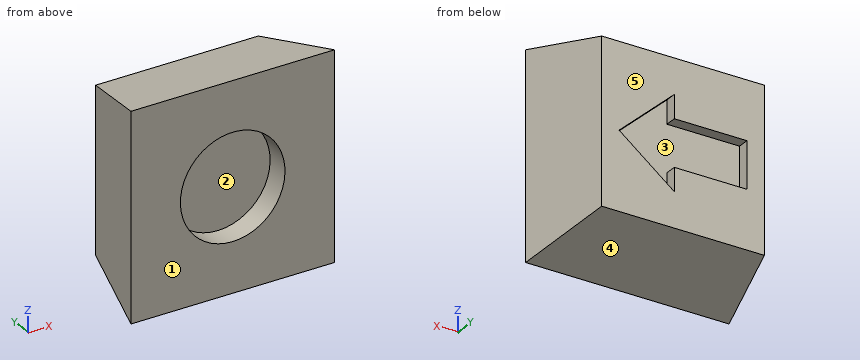
from build123d import *

# Parameters (mm, degrees)
SKETCH1_W           = 7
SKETCH1_H           = 7
BOSS_EXTRUDE1_DEPTH = 3
CUT_EXTRUDE1_DEPTH  = 7
CUT_EXTRUDE2_DEPTH  = 11
SKETCH4_R           = 1.8
CUT_EXTRUDE3_DEPTH  = 0.8
SKETCH5_W           = 2.5
SKETCH5_H           = 1.6
CUT_EXTRUDE4_DEPTH  = 0.4


with BuildPart() as part:
    # Sketch1 → Boss-Extrude1 (new body)
    with BuildSketch(Plane(origin=(0, 0, 0), x_dir=(1, 0, 0), z_dir=(0, 1, 0))):
        with Locations((3.5, 3.5)):
            Rectangle(SKETCH1_W, SKETCH1_H)
    extrude(amount=BOSS_EXTRUDE1_DEPTH)

    # Sketch2 → Cut-Extrude1 (cut)
    with BuildSketch(Plane.XY):
        Polygon((0, 0), (0.7, 3), (0, 3), align=None)
        Polygon((7, 0), (6.3, 3), (7, 3), align=None)
    extrude(amount=-CUT_EXTRUDE1_DEPTH, mode=Mode.SUBTRACT)

    # Sketch3 → Cut-Extrude2 (cut)
    with BuildSketch(Plane(origin=(0, 0, 0), x_dir=(0, 0, -1), z_dir=(1, 0, 0))):
        Polygon((0, 0), (0.7, 3), (0, 3), align=None)
        Polygon((7, 3), (6.3, 3), (7, 0), align=None)
    extrude(amount=CUT_EXTRUDE2_DEPTH, mode=Mode.SUBTRACT)

    # Sketch4 → Cut-Extrude3 (cut)
    with BuildSketch(Plane.XZ):
        with Locations(Location((3.5, -3.5, 0), (0, 0, 270))):
            Circle(SKETCH4_R)
    extrude(amount=-CUT_EXTRUDE3_DEPTH, mode=Mode.SUBTRACT)

    # Sketch5 → Cut-Extrude4 (cut)
    with BuildSketch(Plane(origin=(0, 3, 0), x_dir=(1, 0, 0), z_dir=(0, 1, 0))):
        with Locations((2.55, 3.5)):
            Rectangle(SKETCH5_W, SKETCH5_H)
        Polygon((3.8, 1.9), (3.8, 2.7), (3.8, 4.3), (3.8, 5.1), (5.7, 3.624818901), align=None)
    extrude(amount=-CUT_EXTRUDE4_DEPTH, mode=Mode.SUBTRACT)


solid = part.part
Read the model definition and answer for the solid it produces. Units are mm, in the model's axes. Face numbers are marked on the shaded views. A direction names the side the tool comes from. Round coordinates to 2 decimals unless told otherwise and drop trailing zeros. Write each loop counter-clockwise with the first axis right and the second up, starting at its lowest first coordinate (ties: lowest second). Pieces come first, ordered by that corner, then holes. Notation, with made-up numbers: (-33.5, 20) - (6.5, 20) arc R25 ccw to (6.5, 41) - close; hole circle Ø9 at (33.5, 18.25). An arc over 180 degrees is marked (long way). One line per question, with ' | ' between items. Start each with the question number.
1. Find the intervals of material crossed by probe 1 along X at (y, z) = (0.3, -4); probe 2 along Z at (x, y) = (2, 0.55); probe 3 along Y at (x, z) = (2.25, -2.5), in increasing order. Write a range as [from, to].
2. Section D-D (x = 5.5) is taken. Determine the outline of the cut face in (y, z), and give its area (3 significant figures).
3. For the marked faces 1 and 2, determine the directions among +Z, -Z, +X, -X, +Y, -Y from which every point of the face is accessible in a straight line to the end or side of a thin tool.
4. Section C-C (y = 0.25) is taken. Determine the outline of the cut face in (x, z).
5. Section A-A (x = 3.5) is taken. Determine the outline of the cut face in (y, z), and give its area (3 significant figures).
6. For a pull along Z with two mould halves and no side action, classify the marked faces 3, 4 and 5 as +Z half, -Z half, draft (parallel to the pull), parting line (faces both ways), or undercut.
7. Section B-B (z = -3.25) is taken. Determine the outline of the cut face in (x, y).
Filled in:
1) probe 1: [0.07, 1.77], [5.23, 6.93] | probe 2: [-6.87, -4.49], [-2.51, -0.13] | probe 3: [0.8, 3]
2) outline: (0, -7) - (3, -6.3) - (3, -3.78) - (2.6, -3.78) - (2.6, -3.44) - (3, -3.44) - (3, -0.7) - (0, 0) - close | area: 18.8 mm²
3) face 1: +Z, -Z, +X, -X, -Y | face 2: -Y
4) outline: (0.06, -6.94) - (6.94, -6.94) - (6.94, -0.06) - (0.06, -0.06) - close; hole circle Ø3.6 at (3.5, -3.5)
5) outline: (0, -7) - (3, -6.3) - (3, -4.3) - (2.6, -4.3) - (2.6, -2.7) - (3, -2.7) - (3, -0.7) - (0, 0) - (0, -1.7) - (0.8, -1.7) - (0.8, -5.3) - (0, -5.3) - close | area: 15.4 mm²
6) face 3: undercut | face 4: -Z half | face 5: draft
7) outline: (0, 0) - (1.72, 0) - (1.72, 0.8) - (5.28, 0.8) - (5.28, 0) - (7, 0) - (6.3, 3) - (5.29, 3) - (5.29, 2.6) - (1.3, 2.6) - (1.3, 3) - (0.7, 3) - close
